from build123d import *

# Parameters (mm, degrees)
F0_W      = 15.83
F0_H      = 7.89
F1_DEPTH  = 3.2
F3_DEPTH  = 1.55
F4_R      = 1.59
F6_DEPTH  = 1.55
F7_R      = 1.59
F8_DEPTH  = 1.55
F9_R      = 1.48
F10_DEPTH = 12.83
F11_T     = -1.57
F12_R     = 1.535
F12_R_2   = 0.765
F13_DEPTH = 1.6


with BuildPart() as f1:
    # F0 (on Front) → F1 (new body)
    with BuildSketch(Plane.XZ):
        with Locations((-28.0223558657, 18.9167669917)):
            Rectangle(F0_W, F0_H)
    extrude(amount=F1_DEPTH)

    # F2 (on face) → F3 (join)
    with BuildSketch(Plane.YZ.offset(-20.1073558657)):
        Polygon((-12.81, 14.9717669917), (-3.2, 14.9717669917), (-3.2, 22.8617669917), align=None)
    extrude(amount=-F3_DEPTH)

    # F4
    f4_edges = [f1.edges().sort_by_distance(p)[0] for p in [
        (-20.882356, -12.81, 14.971767),
    ]]
    fillet(f4_edges, radius=F4_R)

    # F5 (on face) → F6 (join)
    with BuildSketch(Plane(origin=(-35.9373558657, 0, 0), x_dir=(0, -1, 0), z_dir=(-1, 0, 0))):
        Polygon((3.2, 22.8617669917), (3.2, 14.9717669917), (12.8218363971, 14.9717669917), align=None)
    extrude(amount=-F6_DEPTH)

    # F7
    f7_edges = [f1.edges().sort_by_distance(p)[0] for p in [
        (-35.162356, -12.821836, 14.971767),
    ]]
    fillet(f7_edges, radius=F7_R)


with BuildPart() as f8:
    # F8 (new): a face of the model
    f8_faces = [f1.part.faces().sort_by_distance(p)[0] for p in [
        (-35.9373558657, -4.069759588, 18.2879557139),
    ]]
    extrude(f8_faces, amount=-F8_DEPTH)


with BuildPart() as f1_1:
    add(f1.part)

    add(f8.part)  # F10 merges F8
    # F9 (on face) → F10 (join)
    with BuildSketch(Plane(origin=(-21.6573558657, 0, 0), x_dir=(0, -1, 0), z_dir=(-1, 0, 0))):
        with Locations((8.367674268, 16.5617669917)):
            Circle(F9_R)
    extrude(amount=F10_DEPTH)

    # F11
    f11_openings = [f1_1.faces().sort_by_distance(p)[0] for p in [
        (-28.022356, 0, 18.916767),
    ]]
    offset(amount=F11_T, openings=f11_openings)

    # F12 (on face) → F13 (join)
    with BuildSketch(Plane(origin=(0, -1.63, 0), x_dir=(-1, 0, 0), z_dir=(0, 1, 0))):
        with Locations((28.0223558657, 18.9167669917)):
            Circle(F12_R)
        with Locations((28.0223558657, 18.9167669917)):
            Circle(F12_R_2, mode=Mode.SUBTRACT)
    extrude(amount=F13_DEPTH)


solid = f1_1.part
Check sheet for the modelled part. Datum: model origin and axes. Units: mm. A direction names the side the tool comes from. Round coordinates to 2 decimals unless told otherwise and drop trailing zeros. Write each loop counter-clockwise with the first axis right and the second up, starting at its lowest first coordinate (ties: lowest second). Pieces come first, ordered by that corner, then holes. Notation, with made-up numbers: (47, 30) - (74, 30) arc R22 cw to (74, 69) - close; hole circle Ø3 at (19, 7.25). An arc over 180 degrees is marked (long way). Return JSON: item names as keys, results as strings.
Q1. Depth check by flat-ended pin: P1, Ø1.4, axis at x = -30.5, z = 18, coming from the +Y side; P2, Ø1.5, axis at x = -27, y = -7.5, coming from the -Z side; P3, Ø1.2, axis at x = -28.02, z = 18.92, coming from the -Y side. Enter the tip coordinate at first touch or a pass-through.
Returned:
{"P1": "stops at y = -1.63", "P2": "stops at z = 15.09", "P3": "stops at y = -3.2"}
Q2. Access from +Z, -Z, +X, -X, +Y, -Y to the whole of each face (thin tool, end or side, straight path). Record for faces 4 (the flat face through (-28, -3.2, 19)), 5 (the flat face through (-28, -1.63, 19)), 6 (the cylindrical face through (-27.93, -8.18, 18.03)), 7 (the flat face through (-35.173, -6.335, 20.291)).
Returned:
{"face 4": "+Z, -Z", "face 5": "+Y", "face 6": "none", "face 7": "+Z, +X, -X, -Y"}
Q3. Cross-section at D-D (x = -21.25). Record the boundary of the cut face in (y, z), then the cut area to 3 significant figures.
Returned:
{"outline": "(-9.38, 17.79) arc R1.59 ccw to (-8.37, 14.97) - (0, 14.97) - (0, 22.86) - (-3.2, 22.86) - close", "area": "59.2 mm²"}
Q4. Cross-section at C-C (z = 19.5). Record the boundary of the cut face in (x, y), then the cut area to 3 significant figures.
Returned:
{"outline": "(-35.94, -7.3) - (-34.39, -7.3) - (-34.39, -3.2) - (-21.66, -3.2) - (-21.66, -7.29) - (-20.11, -7.29) - (-20.11, 0) - (-21.68, 0) - (-21.68, -1.63) - (-26.6, -1.63) - (-26.6, -0.03) - (-27.53, -0.03) - (-27.53, -1.63) - (-28.52, -1.63) - (-28.52, -0.03) - (-29.44, -0.03) - (-29.44, -1.63) - (-34.37, -1.63) - (-34.37, 0) - (-35.94, 0) - close", "area": "45.6 mm²"}
Q5. Cross-section at B-B (x = -29.25). Record the boundary of the cut face in (y, z).
Returned:
{"outline": "circle Ø2.96 at (-8.37, 16.56); (-3.2, 14.97) - (0, 14.97) - (0, 16.54) - (-1.63, 16.54) - (-1.63, 18) - (-0.03, 18) - (-0.03, 19.84) - (-1.63, 19.84) - (-1.63, 21.29) - (0, 21.29) - (0, 22.86) - (-3.2, 22.86) - close"}
Q6. Draft check along X on faces 1 (the flat face through (-35.937, -4, 18)), 2 (the cylindrical face through (-20.893, -9.855, 16)), 3 (the flat face through (-27, -0.03, 19)). Enter one of: released by +X, released by -X, zero draft, split by the parting line, or undercut.
Returned:
{"face 1": "released by -X", "face 2": "zero draft", "face 3": "undercut"}
Q7. Cross-section at A-A (y = -4.25). Record the boundary of the cut face in (x, z).
Returned:
{"outline": "(-35.94, 14.97) - (-34.39, 14.97) - (-34.39, 22) - (-35.94, 22) - close; (-21.66, 14.97) - (-20.11, 14.97) - (-20.11, 22) - (-21.66, 22) - close"}
Q8. Scan lines: L1, parallel to X at y = -1, z = 20.5; L2, parallel to Z at x = -30.25, y = -1; L3, parallel to Y at x = -31.25, z = 22.5. Record each from-to range of solid material in increasing order. Write a range as from..to.
Returned:
{"L1": "x = -35.94..-34.37, -21.68..-20.11", "L2": "z = 14.97..16.54, 21.29..22.86", "L3": "y = -3.2..0"}
